The listing builds one solid part. Answer for the finished solid, in the listing's coordinates (mm). A direction names the side the tool comes from. Coordinates: 2 decimals unless noted, no trailing zeros. Order: outer loops, then holes, each group sorted by start corner. A loop starts at its lowest first (then second) coordinate and runs counter-clockwise, first axis right, second up. Notation, with made-up numbers: (76.25, -40) - (127.25, -40) arc R14 ccw to (127.25, -29) - close; hole circle Ø4 at (-33.75, -25). An arc over 180 degrees is marked (long way). Use a Markdown table: item, result. Add a question column.
Item 1: The part is cut by section D-D, the plane z = -6.5. Give the vertices of the cut face in (x, y).
Item 2: The mould has two halves that part along X. Classify faces 1 (the flat face through (17, 1, -20)), 2 (the flat face through (2, 6, -1)), 3 (the flat face through (4, 2, -22)): released by +X, released by -X, zero draft, split by the parting line, or undercut.
Item 3: The part is cut by section A-A, the plane z = -2.1. Give the vertices of the cut face in (x, y).
Item 4: For faces 4 (the flat face through (3, 6, -20)), 5 (the flat face through (1, 6, -20)), 6 (the flat face through (2, 6, -39.4)), 7 (the flat face through (8.93, 2.84, -18.51)), determine the directions among +Z, -Z, +X, -X, +Y, -Y from which every point of the face is accessible in a straight line to the end or side of a thin tool.
Item 5: The part is cut by section C-C, the plane x = 2.25. Give the vertices of the cut face in (y, z), then the cut area to 3 significant figures.
Item 6: Flat-ended cylindrical pins translate along their axes: P1, Ø1.6, axis at x = 1.5, y = 7.5, coming from the -Z side; P2, Ø5, axis at y = 6.5, z = -30.5, coming from the +X side; P3, Ø1.5, axis at x = 7.5, z = -4.5, coming from the +Y side; P4, Ø3, axis at y = 2, z = -32.5, coming from the +X side. Find the tip coordinate at first contact, or state that the pin passes through.
Item 7: The part is cut by section B-B, the plane y = 4.5. Give the vertices of the cut face in (x, z).
Item 8: Find the intervals of material crossed by line 1 along X through (y, z) = (3.25, -22.5); line 2 along X through (y, z) = (5.5, -22); line 3 along X through (y, z) = (0.6, -38.3), in increasing order.
from build123d import *

# Parameters (mm, degrees)
SKETCH1_W           = 17
SKETCH1_H           = 40.4
BOSS_EXTRUDE1_DEPTH = 1.44
SKETCH2_R           = 1.6
CUT_EXTRUDE1_DEPTH  = 1.44
SKETCH3_W           = 10
SKETCH3_H           = 8
BOSS_EXTRUDE2_DEPTH = 1.89
CHAMFER1_SIZE       = 1
SKETCH4_W           = 2
SKETCH4_H           = 38.4
SKETCH4_W_2         = 1
SKETCH4_H_2         = 10.4
BOSS_EXTRUDE3_DEPTH = 8.5


with BuildPart() as part:
    # Sketch1 → Boss-Extrude1 (new body)
    with BuildSketch(Plane(origin=(0, 0, 0), x_dir=(1, 0, 0), z_dir=(0, 1, 0))):
        with Locations((8.5, 20.2)):
            Rectangle(SKETCH1_W, SKETCH1_H)
    extrude(amount=BOSS_EXTRUDE1_DEPTH)

    # Sketch2 → Cut-Extrude1 (cut)
    with BuildSketch(Plane(origin=(0, 1.44, 0), x_dir=(1, 0, 0), z_dir=(0, 1, 0))):
        with Locations(Location((14.9, 38.3, 0), (0, 0, 270))):
            Circle(SKETCH2_R)
        with Locations(Location((14.9, 2.1, 0), (0, 0, 270))):
            Circle(SKETCH2_R)
    extrude(amount=-CUT_EXTRUDE1_DEPTH, mode=Mode.SUBTRACT)

    # Sketch3 → Boss-Extrude2 (add)
    with BuildSketch(Plane(origin=(0, 1.44, 0), x_dir=(1, 0, 0), z_dir=(0, 1, 0))):
        with Locations((9, 22)):
            Rectangle(SKETCH3_W, SKETCH3_H)
    extrude(amount=BOSS_EXTRUDE2_DEPTH)

    # Chamfer1
    chamfer1_edges = [part.edges().sort_by_distance(p)[0] for p in [
        (9, 3.33, -18),
        (9, 3.33, -26),
    ]]
    chamfer(chamfer1_edges, length=CHAMFER1_SIZE)

    # Sketch4 → Boss-Extrude3 (add)
    with BuildSketch(Plane(origin=(0, 1.44, 0), x_dir=(1, 0, 0), z_dir=(0, 1, 0))):
        with Locations((2, 20.2)):
            Rectangle(SKETCH4_W, SKETCH4_H)
        with Locations((15.5, 20.2)):
            Rectangle(SKETCH4_W_2, SKETCH4_H_2)
    extrude(amount=BOSS_EXTRUDE3_DEPTH)


solid = part.part
Solution:
| question | item | result |
|---|---|---|
| 1 | outline | (0, 0) - (17, 0) - (17, 1.44) - (3, 1.44) - (3, 9.94) - (1, 9.94) - (1, 1.44) - (0, 1.44) - close |
| 2 | face 1 | released by +X |
| 2 | face 2 | zero draft |
| 2 | face 3 | undercut |
| 3 | outline | (0, 0) - (13.3, 0) - (13.3, 1.44) - (3, 1.44) - (3, 9.94) - (1, 9.94) - (1, 1.44) - (0, 1.44) - close; (16.5, 0) - (17, 0) - (17, 1.44) - (16.5, 1.44) - close |
| 4 | face 4 | +Z, -Z, +Y |
| 4 | face 5 | +Z, -Z, -X, +Y |
| 4 | face 6 | -Z, +X, -X, +Y |
| 4 | face 7 | +Z, +Y |
| 5 | outline | (0, -40.4) - (1.44, -40.4) - (1.44, -39.4) - (9.94, -39.4) - (9.94, -1) - (1.44, -1) - (1.44, 0) - (0, 0) - close |
| 5 | area | 385 mm2 |
| 6 | P1 | stops at z = -39.4 |
| 6 | P2 | stops at x = 3 |
| 6 | P3 | stops at y = 1.44 |
| 6 | P4 | stops at x = 17 |
| 7 | outline | (1, -39.4) - (3, -39.4) - (3, -1) - (1, -1) - close; (15, -25.4) - (16, -25.4) - (16, -15) - (15, -15) - close |
| 8 | line 1 | x = 1 to 3, 4 to 14, 15 to 16 |
| 8 | line 2 | x = 1 to 3, 15 to 16 |
| 8 | line 3 | x = 0 to 13.3, 16.5 to 17 |
